from build123d import *

# Parameters (mm, degrees)
EXTRUDE_1_DEPTH     = 16
EXTRUDE_2_DEPTH     = 2
FILLET_1_R          = 2
EXTRUDE_3_DEPTH     = 2
SKETCH_4_R          = 2.5
CUT_EXTRUDE_1_DEPTH = 16
SKETCH_5_R          = 2.5
CUT_EXTRUDE_2_DEPTH = 16


with BuildPart() as part:
    # 草图1 → 凸台-拉伸1 (new body)
    with BuildSketch(Plane(origin=(0, 0, 0), x_dir=(0, 0, -1), z_dir=(1, 0, 0))):
        Polygon((0, 0), (17, 0), (17, 17), (15, 17), (15, 2), (0, 2), align=None)
    extrude(amount=EXTRUDE_1_DEPTH)

    # 草图2 → 凸台-拉伸2 (add)
    with BuildSketch(Plane.XY.offset(-15)):
        with BuildLine():
            Line((0, 17), (16, 17))
            ThreePointArc((16, 17), (8, 25), (0, 17))
        make_face()
    extrude(amount=-EXTRUDE_2_DEPTH)

    # 圆角1
    fillet_1_edges = [part.edges().sort_by_distance(p)[0] for p in [
        (8, 2, -15),
    ]]
    fillet(fillet_1_edges, radius=FILLET_1_R)

    # 草图3 → 凸台-拉伸3 (add)
    with BuildSketch(Plane(origin=(0, 2, 0), x_dir=(1, 0, 0), z_dir=(0, 1, 0))):
        with BuildLine():
            Line((0, 0), (16, 0))
            ThreePointArc((16, 0), (8, -8), (0, 0))
        make_face()
    extrude(amount=-EXTRUDE_3_DEPTH)

    # 草图4 → 切除-拉伸1 (cut)
    with BuildSketch(Plane.XY.offset(-15)):
        with Locations((8, 17)):
            Circle(SKETCH_4_R)
    extrude(amount=-CUT_EXTRUDE_1_DEPTH, mode=Mode.SUBTRACT)

    # 草图5 → 切除-拉伸2 (cut)
    with BuildSketch(Plane(origin=(0, 2, 0), x_dir=(1, 0, 0), z_dir=(0, 1, 0))):
        with Locations(Location((8, 0, 0), (0, 0, 270))):
            Circle(SKETCH_5_R)
    extrude(amount=-CUT_EXTRUDE_2_DEPTH, mode=Mode.SUBTRACT)


solid = part.part
Source: CAD feature listing. Evaluate the final solid. Frame: model axes, mm. A direction names the side the tool comes from. Coordinates: 2 decimals unless noted, no trailing zeros. Loops run counter-clockwise (first coordinate to the right, second up) from the corner with the lowest first, then second, coordinate; pieces in that order, holes last. Notation, with made-up numbers: (24, -31) - (49, -31) arc R17 cw to (49, -27) - close; hole circle Ø10 at (61.25, 75). An arc over 180 degrees is marked (long way). One line per item, written item: value. Start each with the question number.
1. Ray query, L1, parallel to Y at x = 8, z = -16; L2, parallel to Y at x = 7, z = -11.5; L3, parallel to Z at x = 7.5, y = 22.5. Return the intervals inside material, ascending.
2. Mould query, pull axis Y, two halves, no side actions, for faces 3 (the cylindrical face through (8, 1, 8)), 4 (the flat face through (8, 0, -5)), 5 (the flat face through (8, 2, -3)), 6 (the cylindrical face through (9.34, 19.11, -15.99)). Classes: pulls with the +Y half, pulls with the -Y half, needs draft (parallel to the pull), parting line crosses it, or undercut.
3. Section D-D (y = 7.75). Return the cut outline in (x, z), and give its area (3 significant figures).
4. Section A-A (x = 8). Return the cut outline in (y, z).
5. Set-up query: faces 1 (the flat face through (0, 1.6, -12.2)), 2 (the flat face through (8, 12, -15)). Return all of +Z, -Z, +X, -X, +Y, -Y with unobstructed straight access to the full face (end or side cutting, diameter ignored); none if empty.
6. Contact query for flat-ended pins moving along their axis: P1, Ø1.5, axis at x = 3.5, y = 5.5, coming from the +Z side; P2, Ø3, axis at x = 4, z = -2.5, coming from the +Y side; P3, Ø12, axis at y = 4.5, z = -4.5, coming from the -X side. Output: stop coordinate, or through.
7. Section C-C (z = -7.5). Return the cut outline in (x, y).
8. Section B-B (x = 12.75). Return the cut outline in (y, z), and give its area (3 significant figures).
Verdict:
1. L1: y = 0 to 14.5, 19.5 to 25
1. L2: y = 0 to 2
1. L3: z = -17 to -15
2. face 3: needs draft
2. face 4: pulls with the -Y half
2. face 5: pulls with the +Y half
2. face 6: undercut
3. outline: (0, -17) - (16, -17) - (16, -15) - (0, -15) - close
3. area: 32.0 mm2
4. outline: (0, -17) - (14.5, -17) - (14.5, -15) - (4, -15) arc R2 cw to (2, -13) - (2, -2.5) - (0, -2.5) - close; (0, 2.5) - (2, 2.5) - (2, 8) - (0, 8) - close; (19.5, -17) - (25, -17) - (25, -15) - (19.5, -15) - close
5. face 1: +Z, -Z, -X, +Y, -Y
5. face 2: +Z, +X, -X, +Y
6. P1: stops at z = -15
6. P2: stops at y = 2
6. P3: stops at x = 0
7. outline: (0, 0) - (16, 0) - (16, 2) - (0, 2) - close
8. outline: (0, -17) - (23.44, -17) - (23.44, -15) - (4, -15) arc R2 cw to (2, -13) - (2, 6.44) - (0, 6.44) - close
8. area: 90.6 mm2
